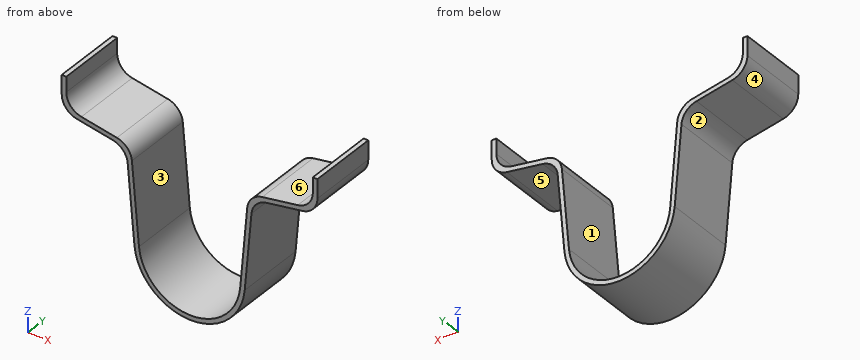
from build123d import *

# Parameters (mm, degrees)
BOSS_EXTRUDE2_DEPTH = 30.48
BOSS_EXTRUDE3_DEPTH = 30.48
CUT_EXTRUDE2_DEPTH  = 87.125730482
FILLET1_R           = 8


with BuildPart() as part:
    # Sketch1 → Boss-Extrude2 (new body)
    with BuildSketch(Plane(origin=(0, 0, 0), x_dir=(1, 0, 0), z_dir=(0, 1, 0))):
        with BuildLine():
            ThreePointArc((-22.169540289, 1.937007843), (0, 22.254), (22.169540289, 1.937007843))
            Line((22.169540289, 1.937007843), (27.396679476, -57.888910388))
            Line((27.396679476, -57.888910388), (29.404298913, -57.888910388))
            Line((29.404298913, -57.888910388), (24.161949769, 2.111089612))
            ThreePointArc((24.161949769, 2.111089612), (0, 24.254), (-24.161949769, 2.111089612))
            Line((-24.161949769, 2.111089612), (-29.404298913, -57.888910388))
            Line((-29.404298913, -57.888910388), (-27.396679476, -57.888910388))
            Line((-27.396679476, -57.888910388), (-22.169540289, 1.937007843))
        make_face()
    extrude(amount=BOSS_EXTRUDE2_DEPTH)

    # Sketch2 → Boss-Extrude3 (add)
    with BuildSketch(Plane(origin=(0, 30.48, 0), x_dir=(1, 0, 0), z_dir=(0, 1, 0))):
        Polygon((-27.656849199, -37.888910388), (-56.013258297, -42.888910388), (-56.013258297, -57.888910388), (-54.013258297, -57.888910388), (-54.013258297, -44.567109651), (-27.837066341, -39.951540757), align=None)
        Polygon((54.013258297, -44.567109651), (27.837066341, -39.951540757), (27.656849199, -37.888910388), (56.013258297, -42.888910388), (56.013258297, -57.888910388), (54.013258297, -57.888910388), align=None)
    extrude(amount=-BOSS_EXTRUDE3_DEPTH)

    # Sketch5 → Cut-Extrude2 (cut, through all)
    with BuildSketch(Plane(origin=(0, 30.48, 0), x_dir=(1, 0, 0), z_dir=(0, 1, 0))):
        Polygon((0, -35.043114897), (-25.798033303, -39.592004218), (-27.396679476, -57.888910388), (27.396679476, -57.888910388), (25.798033303, -39.592004218), align=None)
        Polygon((-25.798033303, -39.592004218), (-27.837066341, -39.951540757), (-29.404298913, -57.888910388), (-27.396679476, -57.888910388), align=None)
        Polygon((27.837066341, -39.951540757), (25.798033303, -39.592004218), (27.396679476, -57.888910388), (29.404298913, -57.888910388), align=None)
    extrude(amount=-CUT_EXTRUDE2_DEPTH, mode=Mode.SUBTRACT)

    # Fillet1
    fillet1_edges = [part.edges().sort_by_distance(p)[0] for p in [
        (-27.656849199, 15.24, 37.888910388),
        (-54.013258297, 15.24, 44.567109651),
        (-56.013258297, 15.24, 42.888910388),
        (54.013258297, 15.24, 44.567109651),
        (27.656849199, 15.24, 37.888910388),
        (56.013258297, 15.24, 42.888910388),
        (-25.798033303, 15.24, 39.592004218),
        (25.798033303, 15.24, 39.592004218),
    ]]
    fillet(fillet1_edges, radius=FILLET1_R)


solid = part.part
Build history of the part. All positions in model axes, mm. Face numbers are marked on the shaded views. A direction names the side the tool comes from. Give positions to 0.01 mm unless a question says otherwise; leave off trailing zeros. Write each loop counter-clockwise with the first axis right and the second up, starting at its lowest first coordinate (ties: lowest second). Pieces come first, ordered by that corner, then holes. Notation, with made-up numbers: (-24.75, -5.5) - (18.25, -5.5) arc R5 cw to (18.25, -1.5) - close; hole circle Ø11 at (50, -17). An arc over 180 degrees is marked (long way). Use one line per item in the form item = value. Start each with the question number.
1. Band-saw the part on D-D on x = 43.5. Write the cut outline in (y, z), plus the area to 3 significant figures.
2. Drop flat-ended pins along their axis: pin 1 Ø5 at (x, y) = (25, 19.5) entering from +Z; pin 2 Ø3 at (y, z) = (6, 6) entering from -X; pin 3 Ø1.5 at (x, y) = (19.5, 6.5) entering from +Z; pin 4 Ø5 at (x, z) = (30, 40.5) entering from -Y. Give the stop position or say it passes through.
3. Band-saw the part on A-A on z = -18.5. Write the cut outline in (x, y), plus the area to 3 significant figures.
4. 3-axis set-ups, long thin cutter, end or side, ignore diameter. For the marked faces 1 and 2: which of +Z, -Z, +X, -X, +Y, -Y reach the whole face in a straight line?
5. Two-plate mould, pull along X, no slides. Class the marked faces 3, 4, 5 and 6: released by +X, released by -X, zero draft, split by the parting line, or undercut.
6. Probe line 1 (X direction, y = 17, z = 25); line 2 (X direction, y = 3.5, z = 54); line 3 (Z direction, x = 0, y = 24.5). List the from-to ranges inside material, lowest first. Write a range as [from, to].
7. Band-saw the part on C-C on x = 13.5. Write the cut outline in (y, z), plus the area to 3 significant figures.
8. Band-saw the part on B-B on z = 47.5. Write the cut outline in (x, y), plus the area to 3 significant figures.
Conclusion:
q1.outline = (0, 40.68) - (30.48, 40.68) - (30.48, 42.71) - (0, 42.71) - close
q1.area = 61.9 mm²
q2.pin_1 = 38.36
q2.pin_2 = -25
q2.pin_3 = -9.23
q2.pin_4 = 0
q3.outline = (-15.68, 0) - (-12.37, 0) - (-12.37, 30.48) - (-15.68, 30.48) - close; (12.37, 0) - (15.68, 0) - (15.68, 30.48) - (12.37, 30.48) - close
q3.area = 202 mm²
q4.face_1 = +Z, +Y, -Y
q4.face_2 = -Z, -X, +Y, -Y
q5.face_3 = undercut
q5.face_4 = released by -X
q5.face_5 = released by +X
q5.face_6 = undercut
q6.line_1 = [-26.53, -24.52], [24.52, 26.53]
q6.line_2 = [-56.01, -54.01], [54.01, 56.01]
q6.line_3 = [-24.25, -22.25]
q7.outline = (0, -20.15) - (30.48, -20.15) - (30.48, -17.69) - (0, -17.69) - close
q7.area = 74.9 mm²
q8.outline = (-55.73, 0) - (-53.06, 0) - (-53.06, 30.48) - (-55.73, 30.48) - close; (53.06, 0) - (55.73, 0) - (55.73, 30.48) - (53.06, 30.48) - close
q8.area = 163 mm²
